```python
from build123d import *

# Parameters (mm, degrees)
SKETCH011_R        = 25.8
PAD007_DEPTH       = 10
SKETCH012_R        = 2.75
POCKET003_DEPTH    = 591.2062275863
POLARPATTERN_COUNT = 3
SKETCH_R           = 35
SKETCH_R_2         = 25.8
PAD_DEPTH          = 20
FILLET_R           = 5
SKETCH013_R        = 3.5
POCKET_DEPTH       = 109.7734133595
POCKET_DEPTH_BACK  = 109.7734133595
FILLET001_R        = 10


with BuildPart() as part:
    # Sketch011 → Pad007 (new body)
    with BuildSketch(Plane.XY):
        Polygon((-54.7724133595, 95.1313972081), (-109.7724133595, -0.1313972081), (-55, -95), (55, -95), (109.7724133595, -0.1313972081), (54.7724133595, 95.1313972081), align=None)
        Circle(SKETCH011_R, mode=Mode.SUBTRACT)
    extrude(amount=PAD007_DEPTH)

    # Sketch012 → Pocket003 (cut, through all)
    with BuildSketch(Plane.XY):
        with Locations((-48.6121593217, 85.8012701892)):
            Circle(SKETCH012_R)
        with Locations((-98.6121593217, -0.8012701892)):
            Circle(SKETCH012_R)
        with Locations((-22.6313972081, 70.8012701892)):
            Circle(SKETCH012_R)
        with Locations((-72.6313972081, -15.8012701892)):
            Circle(SKETCH012_R)
        Polygon((-62.2724133595, 82.1410161514), (-50.6217782649, 52.3205080757), (-70.6217782649, 17.6794919243), (-102.2724133595, 12.8589838486), align=None)
    pocket003 = extrude(amount=POCKET003_DEPTH, mode=Mode.SUBTRACT)

    # PolarPattern: Pocket003 ×3 about axis
    polarpattern_axis = Axis((0, 0, 0), (0, 0, 1))
    for i in range(1, POLARPATTERN_COUNT):
        add(pocket003.rotate(polarpattern_axis, i * 360 / POLARPATTERN_COUNT), mode=Mode.SUBTRACT)

    # Sketch (on Face5 of PolarPattern) → Pad (join)
    with BuildSketch(Plane.XY.offset(10)):
        Circle(SKETCH_R)
        Circle(SKETCH_R_2, mode=Mode.SUBTRACT)
    extrude(amount=PAD_DEPTH)

    # Fillet
    fillet_edges = [part.edges().sort_by_distance(p)[0] for p in [
        (-35, 0, 10),
        (-35, 0, 30),
    ]]
    fillet(fillet_edges, radius=FILLET_R)

    # Sketch013 (on DatumPlane) → Pocket (cut, two sides)
    with BuildSketch(Plane(origin=(0, 0, 15), x_dir=(0, 0, -1), z_dir=(1, 0, 0))) as pocket_sk:
        with Locations((-5, 0)):
            Circle(SKETCH013_R)
    extrude(amount=-POCKET_DEPTH, mode=Mode.SUBTRACT)
    extrude(pocket_sk.sketch, amount=POCKET_DEPTH_BACK, mode=Mode.SUBTRACT)

    # Fillet001
    fillet001_edges = [part.edges().sort_by_distance(p)[0] for p in [
        (20, -70, 5),
        (-20, -70, 5),
        (50.621778, 52.320508, 5),
        (70.621778, 17.679492, 5),
        (-50.621778, 52.320508, 5),
        (-70.621778, 17.679492, 5),
    ]]
    fillet(fillet001_edges, radius=FILLET001_R)


solid = part.part
```
For this review, take the finished solid that the model builds, in its own axes (mm). A direction names the side the tool comes from. Coordinates: 2 decimals unless noted, no trailing zeros. Loops run counter-clockwise (first coordinate to the right, second up) from the corner with the lowest first, then second, coordinate; pieces in that order, holes last.
1. Add section B-B, the plane z = 20. Give the boundary of the cut face in (x, y).
2. Add section A-A, the plane x = 0. Give the boundary of the cut face in (y, z), then the cut area to 3 significant figures.
3. For faces 4 (the cylindrical face through (32.33, -13.41, 19.93)), 5 (the flat face through (0, -70, 5)), 6 (the flat face through (-57.391, 69.647, 4.93)), list the 3-axis set-ups (+Z, -Z, +X, -X, +Y, -Y) from which the entire face can be reached by the end or side of a thin tool; tool diameter is ignored.
4. Insertion check: P1, Ø3, axis at x = 5.5, y = 32, coming from the +Z side; P2, Ø5, axis at x = -50, y = -55, coming from the -Z side; P3, Ø6.5, axis at x = -22.63, y = 70.8, coming from the -Z side; P4, Ø9, axis at x = -48.61, y = 85.8, coming from the +Z side. Each pin has a flat end and moves straight along its axis. Give the tip position at first contact, or say it passes through.
5. Add section C-C, the plane y = -55. Give the boundary of the cut face in (x, z).
6. Mouldability with a two-part tool opening along Z and no side actions: class faces 1 (the cylindrical face through (71.29, 18.55, 5.07)), 2 (the cylindrical face through (-30.21, 1.05, 16.66)), 3 (the flat face through (13.2, 22.4, 30)) as +Z half, -Z half, draft (parallel to the pull), parting line (faces both ways), or undercut.
7. For line 1 (Y direction, x = -50, z = 6); line 2 (Y direction, x = 0, z = 17.5); line 3 (Z direction, x = -41.5, y = -34.5), list the stretches that pass through material, from the lowest coordinate up.
8. Add section D-D, the plane y = -85. Give the boundary of the cut face in (x, z), then the cut area to 3 significant figures.
Result:
1. outline: (-34.82, -3.5) arc R35 ccw to (34.82, -3.5) - (25.56, -3.5) arc R25.8 cw to (-25.56, -3.5) - close; (-34.82, 3.5) - (-25.56, 3.5) arc R25.8 cw to (25.56, 3.5) - (34.82, 3.5) arc R35 ccw to start
2. outline: (-70, 0) - (-25.8, 0) - (-25.8, 30) - (-30, 30) arc R5 ccw to (-35, 25) - (-35, 15) arc R5 cw to (-40, 10) - (-70, 10) - close; (25.8, 0) - (95.13, 0) - (95.13, 10) - (40, 10) arc R5 cw to (35, 15) - (35, 25) arc R5 ccw to (30, 30) - (25.8, 30) - close
2. area: 1,500 mm2
3. face 4: +Z
3. face 5: +Z, -Z, -Y
3. face 6: +Z, -Z, -X
4. P1: stops at z = 29.91
4. P2: passes through
4. P3: stops at z = 0
4. P4: stops at z = 10
5. outline: (-78.09, 0) - (-52.75, 0) - (-52.75, 10) - (-78.09, 10) - close; (-47.25, 0) - (47.25, 0) - (47.25, 10) - (-47.25, 10) - close; (52.75, 0) - (78.09, 0) - (78.09, 10) - (52.75, 10) - close
6. face 1: draft
6. face 2: undercut
6. face 3: +Z half
7. line 1: y = -95 to -87.75, -82.25 to -57.75, -52.25 to 83.43, 88.18 to 95.13
7. line 2: y = -35 to -25.8, 25.8 to 35
7. line 3: z = 0 to 10
8. outline: (-60.77, 0) - (-52.75, 0) - (-52.75, 10) - (-60.77, 10) - close; (-47.25, 0) - (-32, 0) - (-32, 10) - (-47.25, 10) - close; (32, 0) - (47.25, 0) - (47.25, 10) - (32, 10) - close; (52.75, 0) - (60.77, 0) - (60.77, 10) - (52.75, 10) - close
8. area: 465 mm2
